CAD build for the part. Positions are in the model's coordinates, mm. A direction names the side the tool comes from. Coordinates: 2 decimals unless noted, no trailing zeros. Loops run counter-clockwise (first coordinate to the right, second up) from the corner with the lowest first, then second, coordinate; pieces in that order, holes last. Notation, with made-up numbers: (16, 43.25) -> (42, 43.25) arc R26 ccw to (42, 70.25) -> close; hole circle Ø10 at (-27, 79.25). An arc over 180 degrees is marked (long way). Write each question's results on one line, items separated by ' | '.
```python
from build123d import *

# Parameters (mm, degrees)
BOSS_EXTRU_1_DEPTH      = 40
ESQUISSE4_R             = 2.5
ENL_V_MAT_EXTRU_2_DEPTH = 80
ESQUISSE6_R             = 6.505119939
ESQUISSE6_R_2           = 6.755806102
ENL_V_MAT_EXTRU_3_DEPTH = 5


with BuildPart() as part:
    # Esquisse2 → Boss.-Extru.1 (new body)
    with BuildSketch(Plane.XY):
        Polygon((0, 0), (0, 60), (-26, 60), align=None)
    extrude(amount=BOSS_EXTRU_1_DEPTH)

    # Esquisse4 → Enlèv. mat.-Extru.2 (cut)
    with BuildSketch(Plane(origin=(0, 0, 0), x_dir=(0, 0, -1), z_dir=(1, 0, 0))):
        with Locations((-29.388047062, 39.440308957)):
            Circle(ESQUISSE4_R)
        with Locations((-10.611952938, 39.440308957)):
            Circle(ESQUISSE4_R)
    extrude(amount=-ENL_V_MAT_EXTRU_2_DEPTH, mode=Mode.SUBTRACT)

    # Esquisse6 → Enlèv. mat.-Extru.3 (cut)
    with BuildSketch(Plane(origin=(0, 0, 0), x_dir=(0, 0, -1), z_dir=(1, 0, 0))):
        with Locations((-29.388047062, 39.440308957)):
            Circle(ESQUISSE6_R)
        with Locations((-10.611952938, 39.440308957)):
            Circle(ESQUISSE6_R_2)
    extrude(amount=-ENL_V_MAT_EXTRU_3_DEPTH, mode=Mode.SUBTRACT)


solid = part.part
```
Q1. Which spindle directions (+Z, -Z, +X, -X, +Y, -Y) get a long thin tool onto all of the face, cutting with end or side? Do faces 1 (the cylindrical face through (-11.49, 41.92, 29.71)), 2 (the flat face through (-5, 36.5, 10.7)). Say none if no direction does.
Results are:
face 1: +X, -X | face 2: +X
Q2. Cut at A-A on z = 11. Write the cut outline in (x, y).
Results are:
outline: (-26, 60) -> (-18.16, 41.91) -> (-5, 41.91) -> (-5, 46.18) -> (0, 46.18) -> (0, 60) -> close; (-16.02, 36.97) -> (0, 0) -> (0, 32.7) -> (-5, 32.7) -> (-5, 36.97) -> close
Q3. Wall check: L1, parallel to Z at x = -4, y = 39.5; L2, parallel to Z at x = -3.75, y = 40; L3, parallel to X at y = 34, z = 4. Give the ranges that are in metal, low to high. Write a range as from..to.
Results are:
L1: 0..3.86, 17.37..22.88, 35.89..40 | L2: 0..3.88, 17.34..22.91, 35.87..40 | L3: -14.73..0
Q4. Cut at D-D on z = 30. Write the cut outline in (x, y).
Results are:
outline: (-26, 60) -> (-18.14, 41.86) -> (-5, 41.86) -> (-5, 45.92) -> (0, 45.92) -> (0, 60) -> close; (-16.04, 37.02) -> (0, 0) -> (0, 32.96) -> (-5, 32.96) -> (-5, 37.02) -> close
Q5. Cut at B-B on y = 38. Write the cut outline in (x, z), and give its area (4 significant figures).
Results are:
outline: (-16.47, 0) -> (0, 0) -> (0, 4.01) -> (-5, 4.01) -> (-5, 8.57) -> (-16.47, 8.57) -> close; (-16.47, 12.66) -> (-5, 12.66) -> (-5, 17.21) -> (0, 17.21) -> (0, 23.04) -> (-5, 23.04) -> (-5, 27.34) -> (-16.47, 27.34) -> close; (-16.47, 31.43) -> (-5, 31.43) -> (-5, 35.73) -> (0, 35.73) -> (0, 40) -> (-16.47, 40) -> close | area: 435.5 mm^2
Q6. Pull direction Y, two halves, no side cores. Call faces 3 (the cylindrical face through (-2.46, 46.14, 11.49)), 4 (the flat face through (-7, 44, 40)), 5 (the flat face through (-13, 30, 20)): +Y half, -Y half, draft (parallel to the pull), parting line (faces both ways), or undercut.
Results are:
face 3: undercut | face 4: draft | face 5: -Y half
Q7. Drop flat-ended pins along their axis: pin 1 (4 mm diameter, centred on y = 39.44, z = 29.39, fed in from +X); pin 2 (8 mm diameter, centred on x = -6, z = 20.5, fed in from -Y); pin 3 (8 mm diameter, centred on y = 39.44, z = 10.61, fed in from -X); pin 4 (21 mm diameter, centred on y = 39.44, z = 29.39, fed in from -X). Give the stop position or say it passes through.
Results are:
pin 1: through | pin 2: y = 4.62 | pin 3: x = -18.82 | pin 4: x = -21.64
Q8. Cut at C-C on x = -3.5. Write the cut outline in (y, z), and give its area (3 significant figures).
Results are:
outline: (8.08, 0) -> (60, 0) -> (60, 40) -> (8.08, 40) -> close; hole circle Ø13.51 at (39.44, 10.61); hole circle Ø13.01 at (39.44, 29.39) | area: 1,800 mm^2
